Model file for the job. Use its own axes, mm. Face numbers are marked on the shaded views. A direction names the side the tool comes from. Coordinates: 2 decimals unless noted, no trailing zeros. Loops run counter-clockwise (first coordinate to the right, second up) from the corner with the lowest first, then second, coordinate; pieces in that order, holes last.
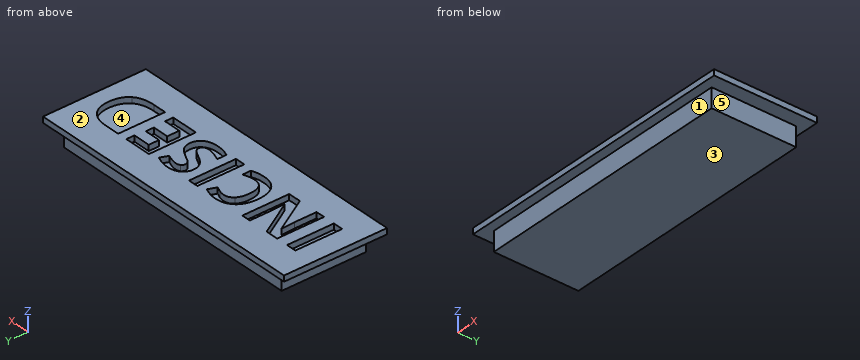
from build123d import *

# Parameters (mm, degrees)
F0_W     = 189.8058950901
F0_H     = 67.760951817
F0_W_2   = 6.5539043493
F0_H_2   = 30.9027749966
F1_DEPTH = 3.81
F2_W     = 171.5631633997
F2_H     = 55.6830503047
F3_DEPTH = 5.08
F4_DEPTH = 12.7


with BuildPart() as f1:
    # F0 (on Top) → F1 (new body)
    with BuildSketch(Plane.XY):
        Rectangle(F0_W, F0_H)
        with Locations((-77.7555048497, -0.57536364)):
            Rectangle(F0_W_2, F0_H_2, mode=Mode.SUBTRACT)
        with BuildLine():
            Line((-39.2876710145, 14.8760238584), (-39.2876710145, -16.0267511383))
            Line((-39.2876710145, -16.0267511383), (-47.6136320609, -16.0267511383))
            Line((-47.6136320609, -16.0267511383), (-61.0596195183, 7.3481646832))
            Line((-61.0596195183, 7.3481646832), (-61.2489996234, 7.3481646832))
            add(Edge.make_bspline(
                [(-61.2489996234, 7.3481646832), (-60.8431851126, 1.1594933937), (-60.8431851126, -1.4850645016)],
                knots=[0, 0, 0, 1, 1, 1], degree=2))
            Line((-60.8431851126, -1.4850645016), (-60.8431851126, -16.0267511383))
            Line((-60.8431851126, -16.0267511383), (-66.7004412183, -16.0267511383))
            Line((-66.7004412183, -16.0267511383), (-66.7004412183, 14.8760238584))
            Line((-66.7004412183, 14.8760238584), (-58.4353523486, 14.8760238584))
            Line((-58.4353523486, 14.8760238584), (-45.0164191918, -8.268930407))
            Line((-45.0164191918, -8.268930407), (-44.8676205378, -8.268930407))
            add(Edge.make_bspline(
                [(-44.8676205378, -8.268930407), (-45.1855085713, -2.2425849218), (-45.1855085713, 0.2464107444)],
                knots=[0, 0, 0, 1, 1, 1], degree=2))
            Line((-45.1855085713, 0.2464107444), (-45.1855085713, 14.8760238584))
            Line((-45.1855085713, 14.8760238584), (-39.2876710145, 14.8760238584))
        make_face(mode=Mode.SUBTRACT)
        with BuildLine():
            add(Edge.make_bspline(
                [(-14.9388003671, 9.2521110963), (-16.6905663387, 9.8642146501), (-18.3814601336, 9.8642146501)],
                knots=[0, 0, 0, 1, 1, 1], degree=2))
            add(Edge.make_bspline(
                [(-18.3814601336, 9.8642146501), (-22.081135757, 9.8642146501), (-24.110208311, 7.0843852512)],
                knots=[0, 0, 0, 1, 1, 1], degree=2))
            add(Edge.make_bspline(
                [(-24.110208311, 7.0843852512), (-26.1392808649, 4.3045558523), (-26.1392808649, -0.6599083297)],
                knots=[0, 0, 0, 1, 1, 1], degree=2))
            add(Edge.make_bspline(
                [(-26.1392808649, -0.6599083297), (-26.1392808649, -10.9946512045), (-18.3814601336, -10.9946512045)],
                knots=[0, 0, 0, 1, 1, 1], degree=2))
            add(Edge.make_bspline(
                [(-18.3814601336, -10.9946512045), (-15.1281804721, -10.9946512045), (-10.5018950491, -9.3713931613)],
                knots=[0, 0, 0, 1, 1, 1], degree=2))
            Line((-10.5018950491, -9.3713931613), (-10.5018950491, -14.8634162073))
            add(Edge.make_bspline(
                [(-10.5018950491, -14.8634162073), (-14.3030243002, -16.4528563746), (-18.996945475, -16.4528563746)],
                knots=[0, 0, 0, 1, 1, 1], degree=2))
            add(Edge.make_bspline(
                [(-18.996945475, -16.4528563746), (-25.7402299293, -16.4528563746), (-29.3113976242, -12.3608933908)],
                knots=[0, 0, 0, 1, 1, 1], degree=2))
            add(Edge.make_bspline(
                [(-29.3113976242, -12.3608933908), (-32.8825653192, -8.268930407), (-32.8825653192, -0.6193268786)],
                knots=[0, 0, 0, 1, 1, 1], degree=2))
            add(Edge.make_bspline(
                [(-32.8825653192, -0.6193268786), (-32.8825653192, 4.2031022246), (-31.12741756, 7.828378521)],
                knots=[0, 0, 0, 1, 1, 1], degree=2))
            add(Edge.make_bspline(
                [(-31.12741756, 7.828378521), (-29.3722698009, 11.4536548174), (-26.0851722635, 13.3846555312)],
                knots=[0, 0, 0, 1, 1, 1], degree=2))
            add(Edge.make_bspline(
                [(-26.0851722635, 13.3846555312), (-22.7980747261, 15.315656245), (-18.3814601336, 15.315656245)],
                knots=[0, 0, 0, 1, 1, 1], degree=2))
            add(Edge.make_bspline(
                [(-18.3814601336, 15.315656245), (-13.8836826391, 15.315656245), (-9.3385601182, 13.1445486123)],
                knots=[0, 0, 0, 1, 1, 1], degree=2))
            Line((-9.3385601182, 13.1445486123), (-11.4487955743, 7.8148513706))
            add(Edge.make_bspline(
                [(-11.4487955743, 7.8148513706), (-13.1870343955, 8.6400075426), (-14.9388003671, 9.2521110963)],
                knots=[0, 0, 0, 1, 1, 1], degree=2))
        make_face(mode=Mode.SUBTRACT)
        with Locations((-0.6507477997, -0.57536364)):
            Rectangle(F0_W_2, F0_H_2, mode=Mode.SUBTRACT)
        with BuildLine():
            add(Edge.make_bspline(
                [(27.0393289865, -2.3406567619), (28.6456780917, -4.4204561297), (28.6456780917, -7.4437742351)],
                knots=[0, 0, 0, 1, 1, 1], degree=2))
            add(Edge.make_bspline(
                [(28.6456780917, -7.4437742351), (28.6456780917, -11.6304272714), (25.6325053491, -14.041641823)],
                knots=[0, 0, 0, 1, 1, 1], degree=2))
            add(Edge.make_bspline(
                [(25.6325053491, -14.041641823), (22.6193326065, -16.4528563746), (17.2558174889, -16.4528563746)],
                knots=[0, 0, 0, 1, 1, 1], degree=2))
            add(Edge.make_bspline(
                [(17.2558174889, -16.4528563746), (12.3048804572, -16.4528563746), (8.5037512062, -14.586109625)],
                knots=[0, 0, 0, 1, 1, 1], degree=2))
            Line((8.5037512062, -14.586109625), (8.5037512062, -8.4988919631))
            add(Edge.make_bspline(
                [(8.5037512062, -8.4988919631), (11.6285229392, -9.8989520253), (13.7962487844, -10.4670923405)],
                knots=[0, 0, 0, 1, 1, 1], degree=2))
            add(Edge.make_bspline(
                [(13.7962487844, -10.4670923405), (15.9639746295, -11.0352326556), (17.7630856273, -11.0352326556)],
                knots=[0, 0, 0, 1, 1, 1], degree=2))
            add(Edge.make_bspline(
                [(17.7630856273, -11.0352326556), (19.9139025345, -11.0352326556), (21.0670921027, -10.2134582712)],
                knots=[0, 0, 0, 1, 1, 1], degree=2))
            add(Edge.make_bspline(
                [(21.0670921027, -10.2134582712), (22.2202816708, -9.3916838869), (22.2202816708, -7.7616622685)],
                knots=[0, 0, 0, 1, 1, 1], degree=2))
            add(Edge.make_bspline(
                [(22.2202816708, -7.7616622685), (22.2202816708, -6.8553431944), (21.7130135324, -6.1451678005)],
                knots=[0, 0, 0, 1, 1, 1], degree=2))
            add(Edge.make_bspline(
                [(21.7130135324, -6.1451678005), (21.2057453939, -5.4349924067), (20.2216452052, -4.7823074018)],
                knots=[0, 0, 0, 1, 1, 1], degree=2))
            add(Edge.make_bspline(
                [(20.2216452052, -4.7823074018), (19.2375450165, -4.129622397), (16.2142269112, -2.6889808837)],
                knots=[0, 0, 0, 1, 1, 1], degree=2))
            add(Edge.make_bspline(
                [(16.2142269112, -2.6889808837), (13.387052486, -1.3565565732), (11.9700834858, -0.1323494657)],
                knots=[0, 0, 0, 1, 1, 1], degree=2))
            add(Edge.make_bspline(
                [(11.9700834858, -0.1323494657), (10.5531144856, 1.0918576419), (9.7076675882, 2.7218792602)],
                knots=[0, 0, 0, 1, 1, 1], degree=2))
            add(Edge.make_bspline(
                [(9.7076675882, 2.7218792602), (8.8622206907, 4.3519008785), (8.8622206907, 6.5230085113)],
                knots=[0, 0, 0, 1, 1, 1], degree=2))
            add(Edge.make_bspline(
                [(8.8622206907, 6.5230085113), (8.8622206907, 10.6284986454), (11.6420500896, 12.9720774452)],
                knots=[0, 0, 0, 1, 1, 1], degree=2))
            add(Edge.make_bspline(
                [(11.6420500896, 12.9720774452), (14.4218794885, 15.315656245), (19.3254714939, 15.315656245)],
                knots=[0, 0, 0, 1, 1, 1], degree=2))
            add(Edge.make_bspline(
                [(19.3254714939, 15.315656245), (21.7333042579, 15.315656245), (23.9213208286, 14.7475159299)],
                knots=[0, 0, 0, 1, 1, 1], degree=2))
            add(Edge.make_bspline(
                [(23.9213208286, 14.7475159299), (26.1093373992, 14.1793756148), (28.4968794377, 13.1445486123)],
                knots=[0, 0, 0, 1, 1, 1], degree=2))
            Line((28.4968794377, 13.1445486123), (26.3866439816, 8.0448129267))
            add(Edge.make_bspline(
                [(26.3866439816, 8.0448129267), (23.9111754658, 9.0593492037), (22.2946809978, 9.4617819269)],
                knots=[0, 0, 0, 1, 1, 1], degree=2))
            add(Edge.make_bspline(
                [(22.2946809978, 9.4617819269), (20.6781865298, 9.8642146501), (19.1158006633, 9.8642146501)],
                knots=[0, 0, 0, 1, 1, 1], degree=2))
            add(Edge.make_bspline(
                [(19.1158006633, 9.8642146501), (17.2558174889, 9.8642146501), (16.2615719374, 8.9984770271)],
                knots=[0, 0, 0, 1, 1, 1], degree=2))
            add(Edge.make_bspline(
                [(16.2615719374, 8.9984770271), (15.267326386, 8.1327394041), (15.267326386, 6.739442917)],
                knots=[0, 0, 0, 1, 1, 1], degree=2))
            add(Edge.make_bspline(
                [(15.267326386, 6.739442917), (15.267326386, 5.873705294), (15.6697591092, 5.2277838643)],
                knots=[0, 0, 0, 1, 1, 1], degree=2))
            add(Edge.make_bspline(
                [(15.6697591092, 5.2277838643), (16.0721918324, 4.5818624347), (16.9480748182, 3.9799042437)],
                knots=[0, 0, 0, 1, 1, 1], degree=2))
            add(Edge.make_bspline(
                [(16.9480748182, 3.9799042437), (17.823957804, 3.3779460527), (21.097528191, 1.8155601861)],
                knots=[0, 0, 0, 1, 1, 1], degree=2))
            add(Edge.make_bspline(
                [(21.097528191, 1.8155601861), (25.4329798813, -0.2608573941), (27.0393289865, -2.3406567619)],
                knots=[0, 0, 0, 1, 1, 1], degree=2))
        make_face(mode=Mode.SUBTRACT)
        Polygon((52.0408846387, -10.6158909944), (52.0408846387, -16.0267511383), (34.2459183406, -16.0267511383), (34.2459183406, 14.8760238584), (52.0408846387, 14.8760238584), (52.0408846387, 9.5057451656), (40.7998226898, 9.5057451656), (40.7998226898, 2.7218792602), (51.263073493, 2.7218792602), (51.263073493, -2.6483994326), (40.7998226898, -2.6483994326), (40.7998226898, -10.6158909944), align=None, mode=Mode.SUBTRACT)
        with BuildLine():
            add(Edge.make_bspline(
                [(79.9406322555, 10.8821327147), (84.1272852918, 6.888241571), (84.1272852918, -0.2811481196)],
                knots=[0, 0, 0, 1, 1, 1], degree=2))
            add(Edge.make_bspline(
                [(84.1272852918, -0.2811481196), (84.1272852918, -7.9104609225), (79.7816882388, -11.9686060304)],
                knots=[0, 0, 0, 1, 1, 1], degree=2))
            add(Edge.make_bspline(
                [(79.7816882388, -11.9686060304), (75.4360911857, -16.0267511383), (67.2386380678, -16.0267511383)],
                knots=[0, 0, 0, 1, 1, 1], degree=2))
            Line((67.2386380678, -16.0267511383), (58.4865717851, -16.0267511383))
            Line((58.4865717851, -16.0267511383), (58.4865717851, 14.8760238584))
            Line((58.4865717851, 14.8760238584), (68.1855385929, 14.8760238584))
            add(Edge.make_bspline(
                [(68.1855385929, 14.8760238584), (75.7539792192, 14.8760238584), (79.9406322555, 10.8821327147)],
                knots=[0, 0, 0, 1, 1, 1], degree=2))
        make_face(mode=Mode.SUBTRACT)
    extrude(amount=F1_DEPTH)

    # F2 (on face) → F3 (cut)
    with BuildSketch(Plane(origin=(0, 0, 0), x_dir=(1, 0, 0), z_dir=(0, 0, -1))):
        Rectangle(F2_W, F2_H)
    extrude(amount=F3_DEPTH, mode=Mode.SUBTRACT)

    # F2 (on face) → F4 (join)
    with BuildSketch(Plane(origin=(0, 0, 0), x_dir=(1, 0, 0), z_dir=(0, 0, -1))):
        Rectangle(F2_W, F2_H)
    extrude(amount=F4_DEPTH)


solid = f1.part
Q1. Flat gauge pins, fed straight in: P1, Ø1, axis at y = 11, z = -6, coming from the +X side; P2, Ø5, axis at x = -78, y = -3, coming from the +Z side; P3, Ø5, axis at x = 45, y = 0.5, coming from the +Z side. Where does each tip first touch, or does it go through?
Answers:
P1: stops at x = 85.78
P2: stops at z = 0
P3: stops at z = 3.81
Q2. Slice it at B-B (x = 43). List the corners of the cut face in (y, z), and give its area (3 significant figures).
Answers:
outline: (-33.88, 0) - (-27.84, 0) - (-27.84, -12.7) - (27.84, -12.7) - (27.84, 0) - (33.88, 0) - (33.88, 3.81) - (14.88, 3.81) - (14.88, 0) - (9.51, 0) - (9.51, 3.81) - (2.72, 3.81) - (2.72, 0) - (-2.65, 0) - (-2.65, 3.81) - (-10.62, 3.81) - (-10.62, 0) - (-16.03, 0) - (-16.03, 3.81) - (-33.88, 3.81) - close
area: 904 mm2
Q3. Mould opens along X. For the marked faces 3, 4 and 5 say: +X half, -X half, draft (parallel to the pull), parting line (faces both ways), or undercut.
Answers:
face 3: draft
face 4: undercut
face 5: +X half
Q4. Which spindle directions (+Z, -Z, +X, -X, +Y, -Y) get a long thin tool onto all of the face, cutting with end or side? Do the marked faces 1 and 2. Say none if no direction does.
Answers:
face 1: -Z, +X, -X, -Y
face 2: +Z, +X, -X, +Y, -Y
Q5. Slice it at C-C (z = -7.25). List the corners of the cut face in (x, y), and give its area (3 significant figures).
Answers:
outline: (-85.78, -27.84) - (85.78, -27.84) - (85.78, 27.84) - (-85.78, 27.84) - close
area: 9,550 mm2
Q6. Slice it at A-A (y = 23.5). List the corners of the cut face in (x, z), and give its area (3 significant figures).
Answers:
outline: (-94.9, 0) - (-85.78, 0) - (-85.78, -12.7) - (85.78, -12.7) - (85.78, 0) - (94.9, 0) - (94.9, 3.81) - (-94.9, 3.81) - close
area: 2,900 mm2
Q7. Drill centre lines: line 1 (Y direction, x = 59, z = 0.75); line 2 (X direction, y = -14, z = -7.25); line 3 (Y direction, x = 13.5, z = 2.5). Where is each one in solid material? Low to high.
Answers:
line 1: y = -33.88 to -16.03, 14.88 to 33.88
line 2: x = -85.78 to 85.78
line 3: y = -33.88 to -16.16, -10.39 to -1.24, 14.17 to 33.88
